The model under review builds one solid part; all positions refer to its coordinate system, in mm. A direction names the side the tool comes from. Round coordinates to 2 decimals unless told otherwise and drop trailing zeros. Order: outer loops, then holes, each group sorted by start corner. A loop starts at its lowest first (then second) coordinate and runs counter-clockwise, first axis right, second up. Notation, with made-up numbers: (5.5, 16) - (26.5, 16) arc R9 cw to (26.5, 25) - close; hole circle Ø5 at (45.25, -9). An arc over 180 degrees is marked (long way). One line per question, with ' | ' between items. Start each with the question number.
Item 1: Insertion check: pin 1 Ø8 at (y, z) = (57, 64) entering from -X; pin 2 Ø12 at (y, z) = (63.5, 201.5) entering from +X; pin 3 Ø10 at (y, z) = (69.5, 174) entering from -X. Each pin has a flat end and moves straight along its axis. Give the tip position at first contact, or say it passes through.
Item 2: Add section A-A on z = 19.5. State the section outline as (x, y) points.
Item 3: Draft analysis for pull direction X (two halves, no side actions). For faces 4 (the face through (31.438, 57.533, 119.552)), 5 (the face through (10.3, 50.2, 213.9)), 6 (the face through (8.896, 49.336, 119.552)), 7 (the face through (31, 62, 242.5)), state which applies: +X half, -X half, draft (parallel to the pull), parting line (faces both ways), or undercut.
Item 4: Add section D-D on x = 32. State the section outline as (y, z) points.
Item 5: Add section B-B on z = 122. State the section outline as (x, y) points, and give its area (3 significant figures).
Item 6: Tool access review of faces 1 (the face through (9.66, 50.6, 116.24)), 2 (the face through (23, 59, 212.5)), 3 (the face through (22.663, 60.376, 14.79)): name each direction out of +Z, -Z, +X, -X, +Y, -Y from which nothing blocks a thin tool from reaching the whole face with its end or side.
Item 7: For L1, parallel to X at y = 68, z = 44; L2, parallel to Y at x = 12.5, z = 223; L3, parallel to X at y = 60.5, z = 220.5, list the stretches that pass through material, from the lowest coordinate up. Write a range as [from, to].
Item 8: Add section C-C on x = 16. State the section outline as (y, z) points.
Autodesk Inventor part; units mm, degrees
ref_plane "Work Plane1" through (0, 0, 121.25) normal (0, 0, -1) x (-1, 0, 0)
ref_plane "YZ Plane" through (0, 0, 0) normal (1, 0, 0) x (0, 1, 0)
ref_plane "XZ Plane" through (0, 0, 0) normal (0, 1, 0) x (-1, 0, 0)
sketch "Sketch1" plane through (0, 0, 0) normal (0, 0, 1) x (1, 0, 0)
  line L0 (10, 0) -> (-1.5, 0)
  line L1 (10, 45.2667) -> (10, 0)
  arc A0 (13.0769, 49.8821) -> (10, 45.2667) centre (15, 45.2667) ccw
  line L2 (54.8615, 67.2923) -> (13.0769, 49.8821)
  line L3 (50.4385, 77.9077) -> (54.8615, 67.2923)
  line L4 (50.4385, 77.9077) -> (29.2692, 69.0872)
  arc A1 (29.2692, 69.0872) -> (-1.5, 22.9333) centre (48.5, 22.9333) ccw
  line L5 (-1.5, 0) -> (-1.5, 22.9333)
  line L6 (29.2692, 69.0872) -> (33.9692, 58.5872)
  line L7 (15, 45.2667) -> (6.8975, 50.6683)
  line L8 (29.2692, 69.0872) -> (50.4077, 77.8949)
  line L9 (50.4077, 77.8949) -> (52.5231, 72.8179)
  line L10 (52.5231, 72.8179) -> (49.2923, 64.9718)
  line L11 (29.8823, 67.7176) -> (50.9846, 76.5103)
  point P0 (0, 0)
  point P1 (10.8397, 48.0402)
  dimension "d2" = 22.9
  dimension "d3" = 5.5
  dimension "d4" = 45
  dimension "d5" = 1.5
extrude "Extrusion1" add sketch "Sketch1" along normal blind 242.5 contours L7 A1 L6 L2 A0 | L6 L11 L9 L10 L2
sketch "Sketch2" plane through (10.8397, 48.0402, 0) normal (-0.5547002, -0.8320503, 0) x (0.8320503, -0.5547002, 0)
  line L0 (-4.738, 0) -> (0, 0)
  line L1 (0, 0) -> (0, 242.5)
  line L2 (-4.738, 242.5) -> (0, 242.5)
  line L3 (-4.738, 0) -> (-4.738, 242.5)
  circle A0 centre (-2.238, 15) radius 1.25
  circle A1 centre (-2.238, 65) radius 1.25
  circle A2 centre (-2.238, 115) radius 1.25
  circle A3 centre (-2.238, 165) radius 1.25
  circle A4 centre (-2.238, 215) radius 1.25
  point P0 (17.6287, 0)
  dimension "d6" = 2.5
  dimension "d7" = 2.5
  dimension "d8" = 15
  dimension "d11" = 50
extrude "Extrusion2" cut sketch "Sketch2" against normal blind 3 contours A0 | A1 | A2 | A3 | A4
sketch "Sketch3" plane through (0, 0, 0) normal (0, 0, -1) x (-1, 0, 0)
  line L0 (-13.0769, 49.8821) -> (-49.2923, 64.9718)
  line L1 (-26.6245, 58.7769) -> (-21.086, 56.4692)
  line L2 (-21.086, 56.4692) -> (-19.9322, 59.2384)
  line L3 (-19.9322, 59.2384) -> (-25.4706, 61.5461)
  line L4 (-25.4706, 61.5461) -> (-26.6245, 58.7769)
  arc A0 (-10.8397, 48.0402) -> (-13.0769, 49.8821) centre (-15, 45.2667) ccw
  line L5 (-6.8975, 50.6683) -> (-10.8397, 48.0402)
  arc A1 (-6.8975, 50.6683) -> (-29.2692, 69.0872) centre (-48.5, 22.9333) ccw
  line L6 (-29.8823, 67.7176) -> (-29.2692, 69.0872)
  line L7 (-50.9846, 76.5103) -> (-29.8823, 67.7176)
  line L8 (-52.5231, 72.8179) -> (-50.9846, 76.5103)
  line L9 (-49.2923, 64.9718) -> (-52.5231, 72.8179)
  line L10 (-13.0769, 49.8821) -> (-49.2923, 64.9718)
  point P0 (0, 0)
  dimension "d20" = 6
  dimension "d21" = 3
  dimension "d22" = 3
  dimension "d32" = 12.7
extrude "Extrusion3" cut sketch "Sketch3" against normal blind 30 contours L4 L3 L2 L1
sketch "Sketch4" plane through (49.2923, 64.9718, 0) normal (0.3846154, -0.9230769, 0) x (0.9230769, 0.3846154, 0)
  line L0 (-29.3068, 0) -> (-23.3068, 0)
  line L1 (-29.3068, 0) -> (-29.3068, 30)
  line L2 (-29.3068, 30) -> (-23.3068, 30)
  line L3 (-23.3068, 0) -> (-23.3068, 30)
  circle A0 centre (-26.3068, 26.4) radius 1.65
  line L4 (-26.3068, 29.7486) -> (-23.4068, 28.0743)
  line L5 (-23.4068, 28.0743) -> (-23.4068, 24.7257)
  line L6 (-23.4068, 24.7257) -> (-26.3068, 23.0514)
  line L7 (-26.3068, 23.0514) -> (-29.2068, 24.7257)
  line L8 (-29.2068, 24.7257) -> (-29.2068, 28.0743)
  line L9 (-29.2068, 28.0743) -> (-26.3068, 29.7486)
  point P0 (-70.4897, 0)
  point P1 (-26.3068, 30)
  dimension "d26" = 3.3
  dimension "d27" = 3.6
  dimension "d28" = 5.8
extrude "Extrusion4" cut sketch "Sketch4" against normal through all contours A0
ref_plane "Work Plane1" through (0, 0, 121.25) normal (0, 0, -1) x (-1, 0, 0)
mirror "Mirror1" about plane through (0, 0, 121.25) normal (0, 0, -1) of "Extrusion4", "Extrusion3"
properties part number "ESQUINA_REDONDEADA_R50"
Determined:
1) pin 1: x = 8.55 | pin 2: x = 51.16 | pin 3: x = 20.71
2) outline: (6.9, 50.67) - (10.84, 48.04) arc R5 cw to (13.08, 49.88) - (49.29, 64.97) - (52.52, 72.82) - (50.98, 76.51) - (29.88, 67.72) - (29.27, 69.09) arc R50 ccw to start; hole (19.93, 59.24) - (21.09, 56.47) - (26.62, 58.78) - (25.47, 61.55) - close
3) face 4: +X half | face 5: undercut | face 6: -X half | face 7: draft
4) outline: (57.77, 0) - (68.6, 0) - (68.6, 242.5) - (57.77, 242.5) - close
5) outline: (6.9, 50.67) - (10.84, 48.04) arc R5 cw to (13.08, 49.88) - (49.29, 64.97) - (52.52, 72.82) - (50.98, 76.51) - (29.88, 67.72) - (29.27, 69.09) arc R50 ccw to start | area: 453 mm2
6) face 1: none | face 2: +Z | face 3: -Z
7) L1: [26.84, 29.76], [30.56, 50.54] | L2: [49.6, 57.63] | L3: [15.5, 22.96], [25.91, 38.56]
8) outline: (51.1, 0) - (60.93, 0) - (60.93, 242.5) - (51.1, 242.5) - close
